Part model, mm, in its own coordinate system. Face numbers are marked on the shaded views. Round coordinates to 2 decimals unless told otherwise and drop trailing zeros. Loops run counter-clockwise (first coordinate to the right, second up) from the corner with the lowest first, then second, coordinate; pieces in that order, holes last. Notation, with made-up numbers: (35.5, 28) -> (53.5, 28) arc R13 ccw to (53.5, 41) -> close; hole circle Ø2 at (67.25, 56). An arc over 180 degrees is marked (long way). Answer as a JSON object with one key per item and string values. Group by question number.
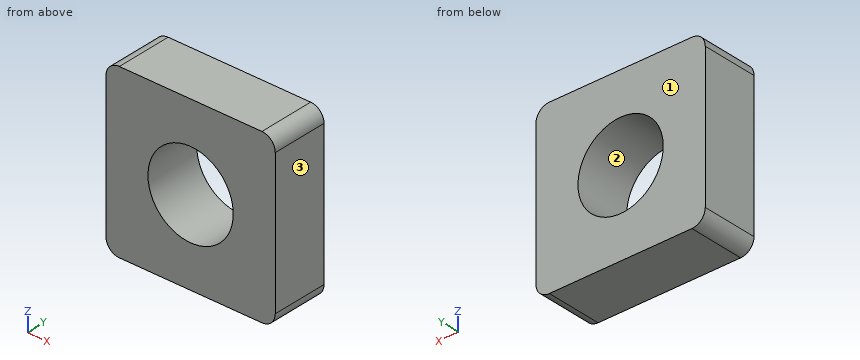
from build123d import *

# Parameters (mm, degrees)
BOSS_EXTRUDE1_DEPTH      = 1.05
BOSS_EXTRUDE1_DEPTH_BACK = 1.05
SKETCH1_R                = 1.6


with BuildPart() as part:
    # Sketch1 → Boss-Extrude1 (new, two sides: drawn at the far end of the back side and taken through both)
    with BuildSketch(Plane(origin=(0, 0, 0), x_dir=(1, 0, 0), z_dir=(0, 1, 0)).offset(-BOSS_EXTRUDE1_DEPTH_BACK)):
        with BuildLine():
            Line((-2.675, 3.175), (2.675, 3.175))
            ThreePointArc((2.675, 3.175), (3.028553391, 3.028553391), (3.175, 2.675))
            Line((3.175, 2.675), (3.175, -2.675))
            ThreePointArc((3.175, -2.675), (3.028553391, -3.028553391), (2.675, -3.175))
            Line((2.675, -3.175), (-2.675, -3.175))
            ThreePointArc((-2.675, -3.175), (-3.028553391, -3.028553391), (-3.175, -2.675))
            Line((-3.175, -2.675), (-3.175, 2.675))
            ThreePointArc((-3.175, 2.675), (-3.028553391, 3.028553391), (-2.675, 3.175))
        make_face()
        with Locations(Location((0, 0, 0), (0, 0, 270))):
            Circle(SKETCH1_R, mode=Mode.SUBTRACT)
    extrude(amount=BOSS_EXTRUDE1_DEPTH + BOSS_EXTRUDE1_DEPTH_BACK)


solid = part.part
Item 1: Band-saw the part on D-D, the plane x = -3. List the corners of the cut face in (y, z).
Item 2: Band-saw the part on B-B, the plane z = 0. List the corners of the cut face in (x, y) (3 decimals), plus the area to 4 significant figures.
Item 3: Band-saw the part on A-A, the plane y = 0.35. List the corners of the cut face in (x, z) (3 decimals), plus the area to 3 significant figures.
Item 4: Band-saw the part on C-C, the plane x = 1. List the corners of the cut face in (y, z) (3 decimals), plus the area to 3 significant figures.
Item 5: Two-plate mould, pull along X, no slides. Class the marked faces 1, 2 and 3: pulls with the +X half, pulls with the -X half, needs draft (parallel to the pull), parting line crosses it, or undercut.
Item 6: Drop flat-ended pins along their axis: pin 1 Ø3 at (x, z) = (-0.5, -0.5) entering from +Y; pin 2 Ø1.9 at (x, z) = (0, 0) entering from +Y. Give the stop position or say it passes through.
Item 7: Drill centre lines: line 1 (X direction, y = -0.4, z = 0) (3 decimals); line 2 (Z direction, x = 0.5, y = -0.4) (3 decimals); line 3 (X direction, y = -0.25, z = 0.75) (3 decimals). Where is each one in solid material? Low to high.
Entries:
{
 "1": {"outline": "(-1.05, -3.05) -> (1.05, -3.05) -> (1.05, 3.05) -> (-1.05, 3.05) -> close"},
 "2": {"outline": "(-3.175, -1.05) -> (-1.6, -1.05) -> (-1.6, 1.05) -> (-3.175, 1.05) -> close; (1.6, -1.05) -> (3.175, -1.05) -> (3.175, 1.05) -> (1.6, 1.05) -> close", "area": "6.615 mm²"},
 "3": {"outline": "(-3.175, -2.675) arc R0.5 ccw to (-2.675, -3.175) -> (2.675, -3.175) arc R0.5 ccw to (3.175, -2.675) -> (3.175, 2.675) arc R0.5 ccw to (2.675, 3.175) -> (-2.675, 3.175) arc R0.5 ccw to (-3.175, 2.675) -> close; hole circle Ø3.2 at (0, 0)", "area": "32.1 mm²"},
 "4": {"outline": "(-1.05, -3.175) -> (1.05, -3.175) -> (1.05, -1.249) -> (-1.05, -1.249) -> close; (-1.05, 1.249) -> (1.05, 1.249) -> (1.05, 3.175) -> (-1.05, 3.175) -> close", "area": "8.09 mm²"},
 "5": {"face 1": "needs draft", "face 2": "undercut", "face 3": "pulls with the +X half"},
 "6": {"pin 1": "y = 1.05", "pin 2": "through"},
 "7": {"line 1": "-3.175 to -1.6, 1.6 to 3.175", "line 2": "-3.175 to -1.52, 1.52 to 3.175", "line 3": "-3.175 to -1.413, 1.413 to 3.175"}
}
